from build123d import *

# Parameters (mm, degrees)
F1_DEPTH       = 45
F2_R           = 2
F3_DEPTH       = 25.001
F4_D           = 5
F4_CBORE_D     = 8.25
F4_CBORE_DEPTH = 4


with BuildPart() as f1:
    # F0 (on Right) → F1 (new body, symmetric)
    with BuildSketch(Plane.YZ):
        Polygon((-25, 0), (0, 0), (0, 15), (-20, 15), (-20, 20), (-25, 20), align=None)
    extrude(amount=F1_DEPTH, both=True)

    # F2 (on face) → F3 (cut, through all)
    with BuildSketch(Plane.XZ.offset(25)):
        with Locations((-37.5, 7.5)):
            Circle(F2_R)
        with Locations((37.5, 7.5)):
            Circle(F2_R)
    extrude(amount=-F3_DEPTH, mode=Mode.SUBTRACT)

    # F4 (through all)
    with Locations(Plane.XZ.offset(25)):
        with Locations((-27.5, 7.5), (27.5, 7.5)):
            CounterBoreHole(F4_D / 2, F4_CBORE_D / 2, F4_CBORE_DEPTH)


solid = f1.part
Work out the finished part from the listing and answer in its coordinate system (mm). A direction names the side the tool comes from. Give positions to 0.01 mm unless a question says otherwise; leave off trailing zeros. Order: outer loops, then holes, each group sorted by start corner. A loop starts at its lowest first (then second) coordinate and runs counter-clockwise, first axis right, second up. Notation, with made-up numbers: (35, 3.5) -> (88, 3.5) arc R25 cw to (88, 31.5) -> close; hole circle Ø4 at (20, -35). An arc over 180 degrees is marked (long way). Answer as a JSON object with one key per item and string values. Group by question number.
1. Section C-C on y = -18.75 is taken. Determine the outline of the cut face in (x, z), plus the area to 3 significant figures.
2. Consider line 1 along Z through (x, y) = (37.5, -6.75); line 2 along Z through (x, y) = (-27.5, -22.1) (3 decimals); line 3 along X through (y, z) = (-22, 8). Determine where each line is inside the solid, lowest interval first. Write a range as [from, to].
3. Section D-D on x = 37.5 is taken. Determine the outline of the cut face in (y, z), plus the area to 3 significant figures.
4. Section A-A on x = -27.5 is taken. Determine the outline of the cut face in (y, z) (3 decimals).
5. A tool of negligible diameter and unlimited length cuts with its end or side. For faces 4 (the cylindrical face through (24.227, -23.028, 4.99)), 5 (the flat face through (1, -13, 0)), 6 (the flat face through (1, -10, 15)), from which of +Z, -Z, +X, -X, +Y, -Y can it reach the whole face along a straight path? Write none if from no direction.
6. Section B-B on z = 7.5 is taken. Determine the outline of the cut face in (x, y) (3 decimals), plus the area to 3 significant figures.
7. The mould has two halves that part along Y. Classify faces 1 (the flat face through (1, -22, 20)), 2 (the flat face through (1, -20, 17)), 3 (the flat face through (-24.8, -21, 7.6)): released by +Y, released by -Y, zero draft, split by the parting line, or undercut.
8. Flat-ended cylindrical pins translate along their axes: pin 1 Ø9 at (x, z) = (-28, 9.5) entering from -Y; pin 2 Ø1 at (x, z) = (26, 5.5) entering from -Y; pin 3 Ø1 at (x, y) = (-8.5, -5) entering from +Z; pin 4 Ø2.5 at (x, z) = (5.5, 17) entering from +Y. Find the tip coordinate at first contact, or state that the pin passes through.
Result sheet:
{
 "1": {"outline": "(-45, 0) -> (45, 0) -> (45, 15) -> (-45, 15) -> close; hole circle Ø4 at (-37.5, 7.5); hole circle Ø5 at (-27.5, 7.5); hole circle Ø5 at (27.5, 7.5); hole circle Ø4 at (37.5, 7.5)", "area": "1,290 mm^2"},
 "2": {"line 1": "z = [0, 5.5], [9.5, 15]", "line 2": "z = [0, 3.375], [11.625, 20]", "line 3": "x = [-45, -39.44], [-35.56, -31.59], [-23.41, 23.41], [31.59, 35.56], [39.44, 45]"},
 "3": {"outline": "(-25, 0) -> (0, 0) -> (0, 5.5) -> (-25, 5.5) -> close; (-25, 9.5) -> (0, 9.5) -> (0, 15) -> (-20, 15) -> (-20, 20) -> (-25, 20) -> close", "area": "300 mm^2"},
 "4": {"outline": "(-25, 0) -> (0, 0) -> (0, 5) -> (-21, 5) -> (-21, 3.375) -> (-25, 3.375) -> close; (-25, 11.625) -> (-21, 11.625) -> (-21, 10) -> (0, 10) -> (0, 15) -> (-20, 15) -> (-20, 20) -> (-25, 20) -> close"},
 "5": {"face 4": "-Y", "face 5": "-Z, +X, -X, +Y, -Y", "face 6": "+Z, +X, -X, +Y"},
 "6": {"outline": "(-45, -25) -> (-39.5, -25) -> (-39.5, 0) -> (-45, 0) -> close; (-35.5, -25) -> (-31.625, -25) -> (-31.625, -21) -> (-30, -21) -> (-30, 0) -> (-35.5, 0) -> close; (-25, -21) -> (-23.375, -21) -> (-23.375, -25) -> (23.375, -25) -> (23.375, -21) -> (25, -21) -> (25, 0) -> (-25, 0) -> close; (30, -21) -> (31.625, -21) -> (31.625, -25) -> (35.5, -25) -> (35.5, 0) -> (30, 0) -> close; (39.5, -25) -> (45, -25) -> (45, 0) -> (39.5, 0) -> close", "area": "1,770 mm^2"},
 "7": {"face 1": "zero draft", "face 2": "released by +Y", "face 3": "released by -Y"},
 "8": {"pin 1": "stops at y = -25", "pin 2": "stops at y = -21", "pin 3": "stops at z = 15", "pin 4": "stops at y = -20"}
}
